The listing builds one solid part. Answer for the finished solid, in the listing's coordinates (mm). Coordinates: 2 decimals unless noted, no trailing zeros. Write each loop counter-clockwise with the first axis right and the second up, starting at its lowest first coordinate (ties: lowest second). Pieces come first, ordered by that corner, then holes. Notation, with made-up numbers: M 4.25,55.5 L 20.25,55.5 A23 ccw 20.25,79.5 Z; hole C 16,49.25 d5. An arc over 180 degrees is marked long. Put each result on its own line as item: value. Start each with the question number.
```python
from build123d import *

# Parameters (mm, degrees)
ESQUISSE1_R        = 1.5
ESQUISSE1_W        = 5
ESQUISSE1_H        = 5
BOSS_EXTRU_1_DEPTH = 2
FILLET1_R          = 5


with BuildPart() as part:
    # Esquisse1 → Boss.-Extru.1 (new body)
    with BuildSketch(Plane.XY):
        Polygon((-10, -15), (-10, 15), (34, 15), (54, 12.5), (54, -12.5), (34, -15), align=None)
        with Locations((-5.5, 0)):
            Circle(ESQUISSE1_R, mode=Mode.SUBTRACT)
        with Locations((49.5, 0)):
            Circle(ESQUISSE1_R, mode=Mode.SUBTRACT)
        with BuildLine():
            Line((4.03758425, 6.699965485), (0, 6.699965485))
            Line((0, 6.699965485), (0, -6.699965485))
            Line((0, -6.699965485), (4.037591434, -6.700034515))
            ThreePointArc((4.037591434, -6.700034515), (4.921479782, -7.066148374), (5.28759897, -7.950034515))
            Line((5.28759897, -7.950034515), (5.28759897, -12.100034515))
            Line((5.28759897, -12.100034515), (29.015776303, -12.100034515))
            Line((29.015776303, -12.100034515), (29.015776303, -8.000038733))
            ThreePointArc((29.015776303, -8.000038733), (29.396536008, -7.080797161), (30.315776345, -6.700034473))
            Line((30.315776345, -6.700034473), (32.315776344, -6.700034473))
            ThreePointArc((32.315776344, -6.700034473), (33.23501504, -7.080795537), (33.615776345, -8.000034132))
            Line((33.615776345, -8.000034132), (33.615776345, -12.100034515))
            Line((33.615776345, -12.100034515), (39.687598777, -12.100034515))
            Line((39.687598777, -12.100034515), (39.687598777, -7.950039613))
            ThreePointArc((39.687598777, -7.950039613), (40.053713738, -7.066152541), (40.937599481, -6.70003437))
            Line((40.937599481, -6.70003437), (44.975197892, -6.70003437))
            Line((44.975197892, -6.70003437), (44.975197892, 6.699965437))
            Line((44.975197892, 6.699965437), (40.9376034, 6.699965437))
            ThreePointArc((40.9376034, 6.699965437), (40.053716981, 7.066080502), (39.68759897, 7.949965701))
            Line((39.68759897, 7.949965701), (39.68759897, 11.987564455))
            Line((39.68759897, 11.987564455), (33.615776432, 11.987564455))
            Line((33.615776432, 11.987564455), (33.615776432, 7.999969389))
            ThreePointArc((33.615776432, 7.999969389), (33.235016597, 7.080728053), (32.315776389, 6.699965495))
            Line((32.315776389, 6.699965495), (30.31577639, 6.699965495))
            ThreePointArc((30.31577639, 6.699965495), (29.396537621, 7.080726637), (29.015776399, 7.999965373))
            Line((29.015776399, 7.999965373), (29.015776399, 11.987564455))
            Line((29.015776399, 11.987564455), (5.28759897, 11.987564455))
            Line((5.28759897, 11.987564455), (5.28759897, 7.949965485))
            ThreePointArc((5.28759897, 7.949965485), (4.921477242, 7.066076805), (4.03758425, 6.699965485))
        make_face(mode=Mode.SUBTRACT)
        with BuildLine():
            ThreePointArc((31.315776387, 9.999965485), (30.315776387, 8.999965485), (31.315776387, 7.999965485))
            ThreePointArc((31.315776387, 7.999965485), (32.315776387, 8.999965485), (31.315776387, 9.999965485))
        make_face(mode=Mode.SUBTRACT)
        with BuildLine():
            ThreePointArc((42.98759897, 8.999965485), (41.98759897, 9.999965485), (40.98759897, 8.999965485))
            ThreePointArc((40.98759897, 8.999965485), (41.98759897, 7.999965485), (42.98759897, 8.999965485))
        make_face(mode=Mode.SUBTRACT)
        with BuildLine():
            ThreePointArc((42.98759897, -9.000034515), (41.98759897, -8.000034515), (40.98759897, -9.000034515))
            ThreePointArc((40.98759897, -9.000034515), (41.98759897, -10.000034515), (42.98759897, -9.000034515))
        make_face(mode=Mode.SUBTRACT)
        with BuildLine():
            ThreePointArc((31.315776387, -8.000034515), (30.315776387, -9.000034515), (31.315776387, -10.000034515))
            ThreePointArc((31.315776387, -10.000034515), (32.315776387, -9.000034515), (31.315776387, -8.000034515))
        make_face(mode=Mode.SUBTRACT)
        with BuildLine():
            ThreePointArc((1.98759897, -9.000034515), (2.98759897, -10.000034515), (3.98759897, -9.000034515))
            ThreePointArc((3.98759897, -9.000034515), (2.98759897, -8.000034515), (1.98759897, -9.000034515))
        make_face(mode=Mode.SUBTRACT)
        with BuildLine():
            ThreePointArc((1.98759897, 8.999965485), (2.98759897, 7.999965485), (3.98759897, 8.999965485))
            ThreePointArc((3.98759897, 8.999965485), (2.98759897, 9.999965485), (1.98759897, 8.999965485))
        make_face(mode=Mode.SUBTRACT)
        with Locations((-5.5, 7.5)):
            Rectangle(ESQUISSE1_W, ESQUISSE1_H, mode=Mode.SUBTRACT)
        with Locations((-5.5, -7.5)):
            Rectangle(ESQUISSE1_W, ESQUISSE1_H, mode=Mode.SUBTRACT)
        with Locations((49.5, 7.5)):
            Rectangle(ESQUISSE1_W, ESQUISSE1_H, mode=Mode.SUBTRACT)
        with Locations((49.5, -7.5)):
            Rectangle(ESQUISSE1_W, ESQUISSE1_H, mode=Mode.SUBTRACT)
    extrude(amount=BOSS_EXTRU_1_DEPTH)

    # Fillet1
    fillet1_edges = [part.edges().sort_by_distance(p)[0] for p in [
        (-10, -15, 1),
        (-10, 15, 1),
        (34, 15, 1),
        (54, 12.5, 1),
        (54, -12.5, 1),
        (34, -15, 1),
    ]]
    fillet(fillet1_edges, radius=FILLET1_R)


solid = part.part
```
1) A cutting plane is placed at D-D on z = 0.65. State how many separate pieces and enclosed holes the cut face has, then the cut area to 3 significant figures.
2) A cutting plane is placed at C-C on y = 6. Write down the section's boundary in (x, z).
3) A cutting plane is placed at B-B on x = 27. Write down the section's boundary in (y, z).
4) Given pin 1 Ø1 at (x, z) = (37.5, 1) entering from -Y (3 decimals); pin 2 Ø6 at (x, y) = (18.5, 7.5) entering from -Z, each flat-ended and moving along its own axis, determine where each tip first touches the part or whether it passes through.
5) A cutting plane is placed at A-A on y = -3. Write down the section's boundary in (x, z), then the cut area to 3 significant figures.
6) Determine the mould class of faces 1 (the face through (22, 14, 0)), 2 (the face through (0, 0, 1)), 3 (the face through (52.715, -11.433, 1.014)) for opening direction X: +X half, -X half, draft (parallel to the pull), parting line (faces both ways), or undercut.
7) Straight lines are drawn through the part: probe 1 along X at (y, z) = (3.5, 1.75); probe 2 along Y at (x, z) = (25, 0.9); probe 3 along Y at (x, z) = (49.5, 1.4). For each, find the intervals that lie inside material, in ascending order.
Answers follow:
1. separate pieces: 1
1. enclosed holes: 13
1. area: 794 mm²
2. outline: M -10,0 L -8,0 L -8,2 L -10,2 Z; M -3,0 L 0,0 L 0,2 L -3,2 Z; M 44.98,0 L 47,0 L 47,2 L 44.98,2 Z; M 52,0 L 54,0 L 54,2 L 52,2 Z
3. outline: M -15,0 L -12.1,0 L -12.1,2 L -15,2 Z; M 11.99,0 L 15,0 L 15,2 L 11.99,2 Z
4. pin 1: stops at y = -14.625
4. pin 2: passes through
5. outline: M -10,0 L 0,0 L 0,2 L -10,2 Z; M 44.98,0 L 54,0 L 54,2 L 44.98,2 Z
5. area: 38.0 mm²
6. face 1: draft
6. face 2: undercut
6. face 3: +X half
7. probe 1: x = -10 to 0, 44.98 to 54
7. probe 2: y = -15 to -12.1, 11.99 to 15
7. probe 3: y = -13.06 to -10, -5 to -1.5, 1.5 to 5, 10 to 13.06
